```python
from build123d import *

# Parameters (mm, degrees)
F0_W      = 20
F0_H      = 25
F0_R      = 8.5
F1_DEPTH  = 10
F2_W      = 1
F2_H      = 6.779089
F3_DEPTH  = 10
F4_R      = 1.6
F5_DEPTH  = 20
F6_W      = 20
F6_H      = 10.463078
F7_DEPTH  = 13.5
F8_W      = 20
F8_H      = 13.5
F9_DEPTH  = 15
F10_R     = 1.6
F11_DEPTH = 14


with BuildPart() as f1:
    # F0 (on Top) → F1 (new body)
    with BuildSketch(Plane.XY):
        Rectangle(F0_W, F0_H)
        with Locations((0, -2.764371)):
            Circle(F0_R, mode=Mode.SUBTRACT)
    extrude(amount=F1_DEPTH)

    # F2 (on face) → F3 (cut)
    with BuildSketch(Plane.XY.offset(10)):
        with Locations((0, 9.110456)):
            Rectangle(F2_W, F2_H)
    extrude(amount=-F3_DEPTH, mode=Mode.SUBTRACT)

    # F4 (on face) → F5 (cut)
    with BuildSketch(Plane(origin=(-10, 0, 0), x_dir=(0, -1, 0), z_dir=(-1, 0, 0))):
        with Locations((-8.5, 5)):
            Circle(F4_R)
    extrude(amount=-F5_DEPTH, mode=Mode.SUBTRACT)

    # F6 (on face) → F7 (join)
    with BuildSketch(Plane.XZ.offset(12.5)):
        with Locations((0, 4.768461)):
            Rectangle(F6_W, F6_H)
    extrude(amount=F7_DEPTH)

    # F8 (on face) → F9 (join)
    with BuildSketch(Plane(origin=(0, 0, -0.463078), x_dir=(1, 0, 0), z_dir=(0, 0, -1))):
        with Locations((0, 19.25)):
            Rectangle(F8_W, F8_H)
    extrude(amount=F9_DEPTH)

    # F10 (on face) → F11 (cut)
    with BuildSketch(Plane(origin=(0, -12.5, 0), x_dir=(-1, 0, 0), z_dir=(0, 1, 0))):
        with Locations((-3, -11.463078)):
            Circle(F10_R)
        with Locations((3, -11.463078)):
            Circle(F10_R)
    extrude(amount=-F11_DEPTH, mode=Mode.SUBTRACT)


solid = f1.part
```
Here's how the part is built. I have some questions about the finished solid (model axes, mm). A direction names the side the tool comes from. Coordinates: 2 decimals unless noted, no trailing zeros. Order: outer loops, then holes, each group sorted by start corner. A loop starts at its lowest first (then second) coordinate and runs counter-clockwise, first axis right, second up.
Item 1: Which directions (+Z, -Z, +X, -X, +Y, -Y) give clear straight access to the entire face, cutting with the end or side of a thin tool? Please do faces 1 (the face through (0, -12.5, -8)), 2 (the face through (3.347, -19.156, -13.025)), 3 (the face through (-0.5, 10, 4)).
Response values:
face 1: -Z, +X, -X, +Y
face 2: +Y, -Y
face 3: +Z, -Z, +Y
Item 2: If we section it at D-D, the plane x = 5.5: List the corners of the cut face in (y, z) for me.
Response values:
outline: (-26, -15.46) - (-12.5, -15.46) - (-12.5, 0) - (-9.25, 0) - (-9.25, 10) - (-26, 10) - close; (3.72, 0) - (12.5, 0) - (12.5, 10) - (3.72, 10) - close; hole circle Ø3.2 at (8.5, 5)
Item 3: I need wall thicknesses on probe 1 along Z at (x, y) = (3, -18.25); probe 2 along Z at (x, y) = (-7, 8.5); probe 3 along Y at (x, z) = (5.75, -9.5). Which ranges of each line are inside material? Lowest first, please.
Response values:
probe 1: z = -15.46 to -13.06, -9.86 to 10
probe 2: z = 0 to 3.4, 6.6 to 10
probe 3: y = -26 to -12.5
Item 4: If we section it at C-C, the plane y = 8.5: List the corners of the cut face in (x, z) for me, then the cut area to 3 significant figures.
Response values:
outline: (-10, 0) - (-0.5, 0) - (-0.5, 3.4) - (-10, 3.4) - close; (-10, 6.6) - (-0.5, 6.6) - (-0.5, 10) - (-10, 10) - close; (0.5, 0) - (10, 0) - (10, 3.4) - (0.5, 3.4) - close; (0.5, 6.6) - (10, 6.6) - (10, 10) - (0.5, 10) - close
area: 129 mm2
Item 5: Thinking about a two-plate mould opening in Z: for faces 4 (the face through (-2.653, -19.156, -13.025)), 5 (the face through (0, -19, -15.463)), 6 (the face through (0, -26, -3)), which applies, pulls with the +Z half, pulls with the -Z half, needs draft (parallel to the pull), parting line crosses it, or undercut?
Response values:
face 4: undercut
face 5: pulls with the -Z half
face 6: needs draft
Item 6: If we section it at A-A, the plane z = 5: Give the number of separate pieces and of enclosed holes in the cut face, then the cut area to 3 significant figures.
Response values:
separate pieces: 3
enclosed holes: 0
area: 475 mm2
Item 7: If we section it at B-B, the plane x = -3: List the corners of the cut face in (y, z) for me, then the cut area to 3 significant figures.
Response values:
outline: (-26, -15.46) - (-12.5, -15.46) - (-12.5, -13.06) - (-26, -13.06) - close; (-26, -9.86) - (-12.5, -9.86) - (-12.5, 0) - (-10.72, 0) - (-10.72, 10) - (-26, 10) - close; (5.19, 0) - (12.5, 0) - (12.5, 10) - (5.19, 10) - close; hole circle Ø3.2 at (8.5, 5)
area: 383 mm2
Item 8: I'm going to push flat-ended pins straight in: pin 1 Ø3 at (y, z) = (8.5, 5) entering from +X; pin 2 Ø5.5 at (y, z) = (8.5, 5) entering from -X. Where does each tip first touch, or does it pass through?
Response values:
pin 1: passes through
pin 2: stops at x = -10
